The figure shows three views and two pictorial views of one solid part (mm, origin at its lowest corner). Answer the questions. Coordinates: 2 decimals unless noted, no trailing zeros. Loops run counter-clockwise (first coordinate to the right, second up) from the corner with the lowest first, then second, coordinate; pieces in that order, holes last. Notation, with made-up numbers: M 77.5,-17 L 133.5,-17 A30 ccw 133.5,22 Z; hole C 32.25,24 d3. An arc over 180 degrees is marked long. Write each question's results on one line, items separated by ' | '.
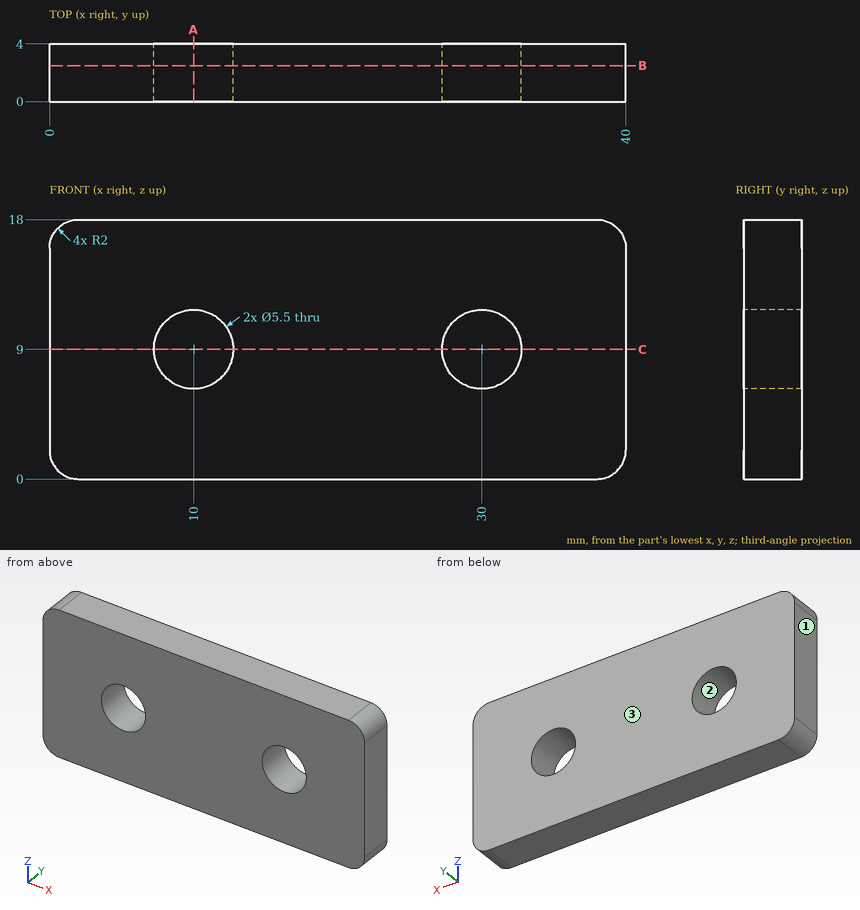
1) Find section C-C, the plane z = 9. Give the vertices of the cut face in (x, y).
Check result:
outline: M 0,0 L 7.25,0 L 7.25,4 L 0,4 Z; M 12.75,0 L 27.25,0 L 27.25,4 L 12.75,4 Z; M 32.75,0 L 40,0 L 40,4 L 32.75,4 Z
2) Straight lines are drawn through the part: probe 1 along X at (y, z) = (2.1, 9); probe 2 along Z at (x, y) = (30, 1.05); probe 3 along X at (y, z) = (2.55, 10.5). For each, find the intervals that lie inside material, in ascending order. Write a range as [from, to].
Check result:
probe 1: [0, 7.25], [12.75, 27.25], [32.75, 40] | probe 2: [0, 6.25], [11.75, 18] | probe 3: [0, 7.7], [12.3, 27.7], [32.3, 40]
3) Find section A-A, the plane x = 10. Give the vertices of the cut face in (y, z).
Check result:
outline: M 0,0 L 4,0 L 4,6.25 L 0,6.25 Z; M 0,11.75 L 4,11.75 L 4,18 L 0,18 Z
4) For a pull along X with two mould halves and no side action, classify the marked faces 1, 2 and 3 as released by +X, released by -X, zero draft, split by the parting line, or undercut.
Check result:
face 1: released by -X | face 2: undercut | face 3: zero draft
5) Find section B-B, the plane y = 2.5. Give the vertices of the cut face in (x, z).
Check result:
outline: M 0,2 A2 ccw 2,0 L 38,0 A2 ccw 40,2 L 40,16 A2 ccw 38,18 L 2,18 A2 ccw 0,16 Z; hole C 10,9 d5.5; hole C 30,9 d5.5
